Could you check a few things on this drawing? It's one solid part, dimensions in mm from its lowest x, y, z. A direction names the side the tool comes from. Round coordinates to 2 decimals unless told otherwise and drop trailing zeros. Write each loop counter-clockwise with the first axis right and the second up, starting at its lowest first coordinate (ties: lowest second). Pieces come first, ordered by that corner, then holes. Notation, with made-up numbers: (12, -8.5) -> (34, -8.5) arc R15 cw to (34, -2.5) -> close; hole circle Ø3 at (30, 75.25). An arc over 180 degrees is marked (long way). Answer in a Markdown table with one row per item. Add a question column.
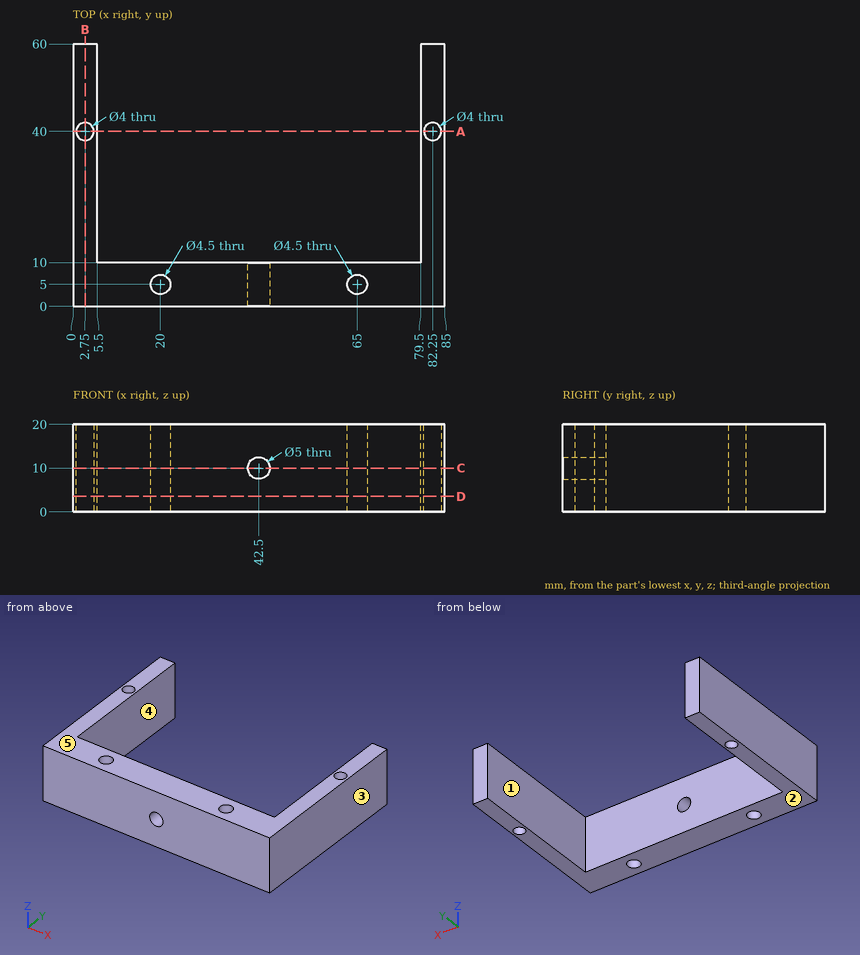
(1) Suppose I cut it at D-D, the plane z = 3.5. Please give me the cut outline in (x, y), then the cut area to 3 significant figures.
(2) For P1, Ø6, axis at x = 42.5, z = 10, coming from the +Y side; P2, Ø3, axis at y = 23, z = 10, coming from the -X side; P3, Ø3, axis at x = 2.75, y = 40, coming from the -Z side, each with a flat end and sliding along its axis, tell me the tip position at first contact or that it passes through.
(3) Suppose I cut it at B-B, the plane x = 2.75. Please give me the cut outline in (y, z), then the cut area to 3 significant figures.
(4) Suppose I cut it at C-C, the plane z = 10. Please give me the cut outline in (x, y), then the cut area to 3 significant figures.
(5) I need wall thicknesses on L1, parallel to X at y = 35, z = 10; L2, parallel to Y at x = 2.75, z = 11; L3, parallel to Y at x = 65, z = 6.5. Which ranges of each line are inside material? Lowest first, please.
(6) On a 3-axis mill with a long thin cutter (end or side, diameter ignored), from which of +Z, -Z, +X, -X, +Y, -Y can I reach the whole of each face in a straight line? I mean the marked faces 1 and 2. Say none if no direction works.
(7) Suppose I cut it at A-A, the plane y = 40. Please give me the cut outline in (x, z).
(8) If we mould it in two halves opening along X, with no side actions, what happens to the marked faces 3, 4 and 5? For each: pulls with the +X half, pulls with the -X half, needs draft (parallel to the pull), parting line crosses it, or undercut.
Response:
| question | item | result |
|---|---|---|
| 1 | outline | (0, 0) -> (85, 0) -> (85, 60) -> (79.5, 60) -> (79.5, 10) -> (5.5, 10) -> (5.5, 60) -> (0, 60) -> close; hole circle Ø4 at (2.75, 40); hole circle Ø4.5 at (20, 5); hole circle Ø4.5 at (65, 5); hole circle Ø4 at (82.25, 40) |
| 1 | area | 1,340 mm² |
| 2 | P1 | y = 10 |
| 2 | P2 | x = 0 |
| 2 | P3 | through |
| 3 | outline | (0, 0) -> (38, 0) -> (38, 20) -> (0, 20) -> close; (42, 0) -> (60, 0) -> (60, 20) -> (42, 20) -> close |
| 3 | area | 1,120 mm² |
| 4 | outline | (0, 0) -> (40, 0) -> (40, 10) -> (5.5, 10) -> (5.5, 60) -> (0, 60) -> close; (45, 0) -> (85, 0) -> (85, 60) -> (79.5, 60) -> (79.5, 10) -> (45, 10) -> close; hole circle Ø4 at (2.75, 40); hole circle Ø4.5 at (20, 5); hole circle Ø4.5 at (65, 5); hole circle Ø4 at (82.25, 40) |
| 4 | area | 1,290 mm² |
| 5 | L1 | 0 to 5.5, 79.5 to 85 |
| 5 | L2 | 0 to 38, 42 to 60 |
| 5 | L3 | 0 to 2.75, 7.25 to 10 |
| 6 | face 1 | +Z, -Z, +Y |
| 6 | face 2 | -Z, +X, -X, +Y, -Y |
| 7 | outline | (0, 0) -> (0.75, 0) -> (0.75, 20) -> (0, 20) -> close; (4.75, 0) -> (5.5, 0) -> (5.5, 20) -> (4.75, 20) -> close; (79.5, 0) -> (80.25, 0) -> (80.25, 20) -> (79.5, 20) -> close; (84.25, 0) -> (85, 0) -> (85, 20) -> (84.25, 20) -> close |
| 8 | face 3 | pulls with the +X half |
| 8 | face 4 | undercut |
| 8 | face 5 | needs draft |
